Source: three-view drawing plus pictorial views. Frame: mm from the lowest corner of the part. A direction names the side the tool comes from. Give positions to 0.01 mm unless a question says otherwise; leave off trailing zeros. Loops run counter-clockwise (first coordinate to the right, second up) from the corner with the lowest first, then second, coordinate; pieces in that order, holes last. Notation, with made-up numbers: (-19.5, -26.75) - (30.5, -26.75) arc R10 cw to (30.5, -11.75) - close; hole circle Ø2 at (51.5, 4.25). An arc over 180 degrees is marked (long way). Write each question's results on one line, items separated by ' | '. Start each with the question number.
(1) Cut plane C-C on x = 32.5. Return the cut outline in (y, z).
(2) Material intervals for line 1 along Y through (x, z) = (2.55, 50); line 2 along X through (y, z) = (33, 41); line 3 along Y through (x, z) = (8.05, 50), sorted ascending. Write a range as [from, to].
(3) Contact query for flat-ended pins moving along their axis: pin 1 (8 mm diameter, centred on x = 76.5, y = 124.5, fed in from +Z); pin 2 (9 mm diameter, centred on y = 13, z = 50, fed in from +X); pin 3 (1.5 mm diameter, centred on x = 38.5, y = 70.5, fed in from -Z); pin 4 (3 mm diameter, centred on y = 52.5, z = 46, fed in from -X). Output: stop coordinate, or through.
(4) Cut plane A-A on y = 13. Return the cut outline in (x, z).
(5) Cut plane B-B on z = 50. Return the cut outline in (x, y).
(6) Reachability of the marked faces 1, 2 and 3 from +Z, -Z, +X, -X, +Y, -Y: full face, straight path, thin tool, end or side. Return the list, or none.
(7) Cut plane D-D on y = 141.5. Return the cut outline in (x, z).
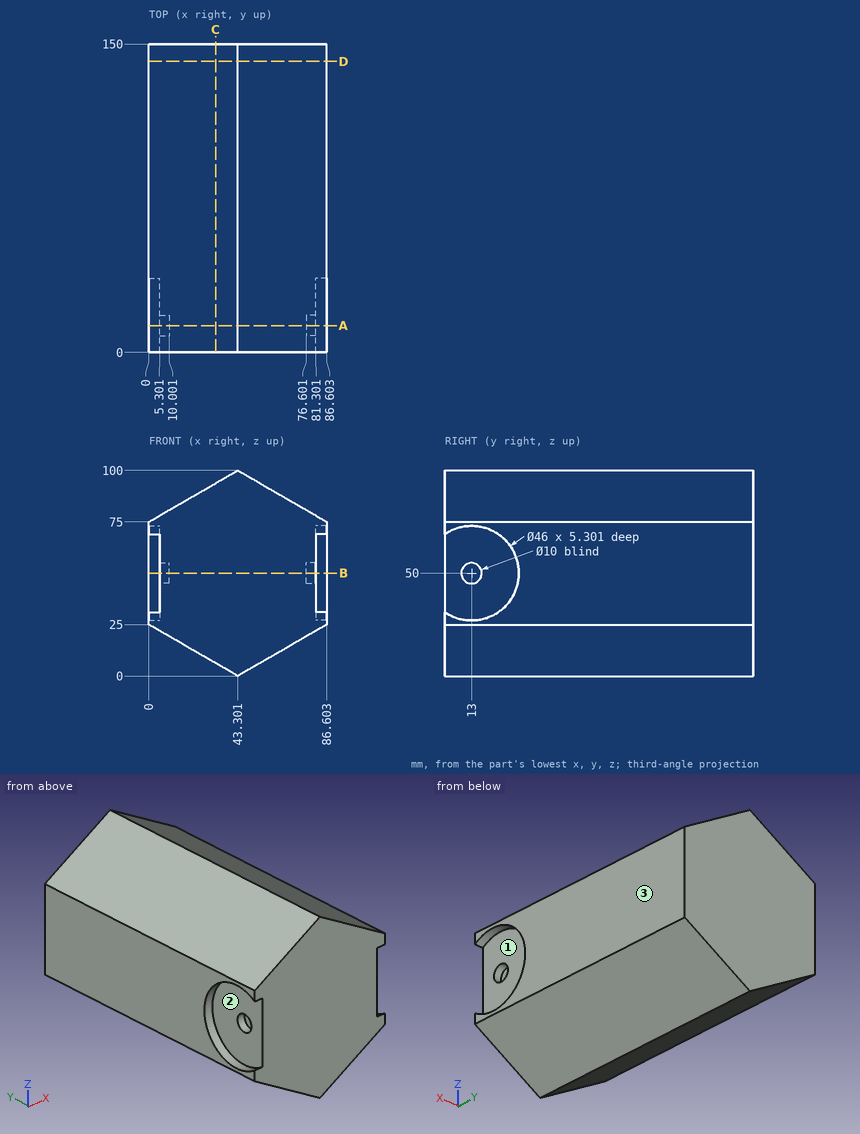
Ans:
1) outline: (0, 6.24) - (150, 6.24) - (150, 93.76) - (0, 93.76) - close
2) line 1: [36, 150] | line 2: [5.3, 81.3] | line 3: [0, 8], [18, 150]
3) pin 1: z = 83.14 | pin 2: x = 76.6 | pin 3: z = 2.34 | pin 4: x = 0
4) outline: (0, 25) - (43.3, 0) - (86.6, 25) - (86.6, 27) - (81.3, 27) - (81.3, 45) - (76.6, 45) - (76.6, 55) - (81.3, 55) - (81.3, 73) - (86.6, 73) - (86.6, 75) - (43.3, 100) - (0, 75) - (0, 73) - (5.3, 73) - (5.3, 55) - (10, 55) - (10, 45) - (5.3, 45) - (5.3, 27) - (0, 27) - close
5) outline: (0, 36) - (5.3, 36) - (5.3, 18) - (10, 18) - (10, 8) - (5.3, 8) - (5.3, 0) - (81.3, 0) - (81.3, 8) - (76.6, 8) - (76.6, 18) - (81.3, 18) - (81.3, 36) - (86.6, 36) - (86.6, 150) - (0, 150) - close
6) face 1: +X | face 2: -X | face 3: +Z, -Z, +X, +Y, -Y
7) outline: (0, 25) - (43.3, 0) - (86.6, 25) - (86.6, 75) - (43.3, 100) - (0, 75) - close
